```python
from build123d import *

# Parameters (mm, degrees)
F0_R      = 31.8731292534
F1_DEPTH  = 50.8
F2_R      = 29.9394143693
F4_DEPTH  = 47.752
F3_R      = 1.3670276657
F3_R_2    = 1.4605226194
F3_R_3    = 1.340090054
F3_R_4    = 1.298632057
F5_DEPTH  = 25.4
F6_DEPTH  = 25.4
F8_START  = 22.098
F8_DEPTH  = 13.208
F10_DEPTH = 67.1801292534
F11_START = -20.828
F11_DEPTH = 14.224
F12_DEPTH = 70.359
F14_START = -12.192
F14_DEPTH = 2.032
F16_START = -6.604
F16_DEPTH = 6.604


with BuildPart() as f1:
    # F0 (on Top) → F1 (new body)
    with BuildSketch(Plane.XY):
        Circle(F0_R)
    extrude(amount=F1_DEPTH)

    # F2 (on face) → F4 (cut)
    with BuildSketch(Plane.XY.offset(50.8)):
        Circle(F2_R)
    extrude(amount=-F4_DEPTH, mode=Mode.SUBTRACT)

    # F3 (on face) → F5 (cut)
    with BuildSketch(Plane(origin=(0, 0, 0), x_dir=(1, 0, 0), z_dir=(0, 0, -1))):
        with Locations((0, 23.9648092538)):
            Circle(F3_R)
        Circle(F3_R_2)
        with Locations((0, -22.0552626997)):
            Circle(F3_R_3)
        with Locations((-19.1909428686, 0)):
            Circle(F3_R_4)
        with Locations((20.7185801119, 0)):
            Circle(F3_R_4)
    extrude(amount=-F5_DEPTH, mode=Mode.SUBTRACT)

    # F3 (on face) → F6 (cut)
    with BuildSketch(Plane(origin=(0, 0, 0), x_dir=(1, 0, 0), z_dir=(0, 0, -1))):
        with Locations((0, 23.9648092538)):
            Circle(F3_R)
        Circle(F3_R_2)
        with Locations((0, -22.0552626997)):
            Circle(F3_R_3)
        with Locations((-19.1909428686, 0)):
            Circle(F3_R_4)
        with Locations((20.7185801119, 0)):
            Circle(F3_R_4)
    extrude(amount=-F6_DEPTH, mode=Mode.SUBTRACT)

    # F7 (on Front) → F8 (join)
    with BuildSketch(Plane.XZ.offset(F8_START)):
        Polygon((11.1125, 24.6736888855), (0, 43.9211034846), (-11.1125, 24.6736888855), align=None)
        Polygon((0, 5.4262742864), (-11.1125, 24.6736888855), (-22.225, 5.4262742864), align=None)
        Polygon((11.1125, 24.6736888855), (-11.1125, 24.6736888855), (0, 5.4262742864), align=None)
        Polygon((22.225, 5.4262742864), (11.1125, 24.6736888855), (0, 5.4262742864), align=None)
    extrude(amount=F8_DEPTH)

    # F9 (on face) → F10 (cut, through all)
    with BuildSketch(Plane.XZ.offset(35.306)):
        Polygon((10.0251361728, 24.6736888855), (-10.0464997813, 24.6736888855), (0, 6.265532691), align=None)
    extrude(amount=-F10_DEPTH, mode=Mode.SUBTRACT)

    # F7 (on Front) → F11 (join)
    with BuildSketch(Plane.XZ.offset(F11_START)):
        Polygon((11.1125, 24.6736888855), (0, 43.9211034846), (-11.1125, 24.6736888855), align=None)
        Polygon((0, 5.4262742864), (-11.1125, 24.6736888855), (-22.225, 5.4262742864), align=None)
        Polygon((11.1125, 24.6736888855), (-11.1125, 24.6736888855), (0, 5.4262742864), align=None)
        Polygon((22.225, 5.4262742864), (11.1125, 24.6736888855), (0, 5.4262742864), align=None)
    extrude(amount=-F11_DEPTH)

    # F9 (on face) → F12 (cut, through all)
    with BuildSketch(Plane.XZ.offset(35.306)):
        Polygon((10.0251361728, 24.6736888855), (-10.0464997813, 24.6736888855), (0, 6.265532691), align=None)
    extrude(amount=-F12_DEPTH, mode=Mode.SUBTRACT)

    # F13 (on face) → F14 (join)
    with BuildSketch(Plane(origin=(0, 35.052, 0), x_dir=(-1, 0, 0), z_dir=(0, 1, 0)).offset(F14_START)):
        Polygon((10.0464997813, 24.6736888855), (-10.0251361728, 24.6736888855), (0, 6.265532691), align=None)
    extrude(amount=-F14_DEPTH)

    # F15 (on face) → F16 (join)
    with BuildSketch(Plane.XZ.offset(35.306).offset(F16_START)):
        Polygon((10.0251361728, 24.6736888855), (-10.0464997813, 24.6736888855), (0, 6.265532691), align=None)
    extrude(amount=-F16_DEPTH)


solid = f1.part
```
CAD build for the part. Positions are in the model's coordinates, mm. A direction names the side the tool comes from. Give positions to 0.01 mm unless a question says otherwise; leave off trailing zeros. Order: outer loops, then holes, each group sorted by start corner. A loop starts at its lowest first (then second) coordinate and runs counter-clockwise, first axis right, second up. Notation, with made-up numbers: M 87,89.5 L 102,89.5 A11 ccw 102,95.5 Z; hole C 67.25,-26.5 d5. An arc over 180 degrees is marked long. Put each result on its own line as item: value. Start each with the question number.
(1) Flat gauge pins, fed straight in: pin 1 Ø12 at (y, z) = (-12, 11) entering from -X; pin 2 Ø3.5 at (x, y) = (0, 22.06) entering from +Z; pin 3 Ø4 at (y, z) = (5, 38) entering from +X. Where does each tip first touch, or does it go through?
(2) Saw through at D-D, the plane y = -9. Write the cut outline in (x, z), then the cut area to 3 significant figures.
(3) Saw through at A-A, the plane y = 0. Write the cut outline in (x, z).
(4) Saw through at C-C, the plane x = -25. Write the cut outline in (y, z).
(5) Which spindle directions (+Z, -Z, +X, -X, +Y, -Y) get a long thin tool onto all of the face, cutting with end or side? Do faces 1 (the flat face through (0, -28.702, 18)), 2 (the flat face through (-13.426, 31.576, 20.666)), 3 (the flat face through (8.5, 24.3, 29.2)). Say none if no direction does.
(6) Mould opens along Y. For faces 4 (the cylindrical face through (14.708, -28.277, 25.044)), 5 (the cylindrical face through (-0.174, 20.727, 1.503)), 6 (the flat face through (0, -32, 24.674)) say: +Y half, -Y half, draft (parallel to the pull), parting line (faces both ways), or undercut.
(7) Saw through at B-B, the plane z = 22. Write the cut outline in (x, y).
(8) Drill centre lines: line 1 along Y through (x, z) = (0, 1); line 2 along X through (y, z) = (-27, 28.5); line 3 along X through (y, z) = (-27.5, 29). Where is each one in solid material? Low to high.
Check result:
1. pin 1: stops at x = -31.3
1. pin 2: stops at z = 43.92
1. pin 3: stops at x = 31.73
2. outline: M -30.58,0 L 30.58,0 L 30.58,50.8 L 28.55,50.8 L 28.55,3.05 L -28.55,3.05 L -28.55,50.8 L -30.58,50.8 Z
2. area: 379 mm2
3. outline: M -31.87,0 L -20.49,0 L -20.49,3.05 L -29.94,3.05 L -29.94,50.8 L -31.87,50.8 Z; M -17.89,0 L -1.46,0 L -1.46,3.05 L -17.89,3.05 Z; M 1.46,0 L 19.42,0 L 19.42,3.05 L 1.46,3.05 Z; M 22.02,0 L 31.87,0 L 31.87,50.8 L 29.94,50.8 L 29.94,3.05 L 22.02,3.05 Z
4. outline: M -19.77,0 L 19.77,0 L 19.77,50.8 L 16.47,50.8 L 16.47,3.05 L -16.47,3.05 L -16.47,50.8 L -19.77,50.8 Z
5. face 1: -Y
5. face 2: +Z, -X, +Y
5. face 3: +Z
6. face 4: parting line
6. face 5: undercut
6. face 6: draft
7. outline: M -12.66,-35.31 L -8.59,-35.31 L -8.59,-28.7 L 8.57,-28.7 L 8.57,-35.31 L 12.66,-35.31 L 12.66,-29.25 A31.87 ccw 12.66,29.25 L 12.66,35.05 L 8.57,35.05 L 8.57,22.86 L -8.59,22.86 L -8.59,35.05 L -12.66,35.05 L -12.66,29.25 A31.87 ccw -12.66,-29.25 Z; hole M -12.66,-27.13 L -12.66,-22.1 L 12.66,-22.1 L 12.66,-27.13 A29.94 ccw 12.66,27.13 L 12.66,20.83 L -12.66,20.83 L -12.66,27.13 A29.94 ccw Z
8. line 1: y = -31.87 to -25.33, -22.6 to -1.46, 1.46 to 20.72, 23.4 to 31.87
8. line 2: x = -16.94 to -12.94, -8.9 to 8.9, 12.94 to 16.94
8. line 3: x = -16.11 to -11.84, -8.61 to 8.61, 11.84 to 16.11
